Check sheet for the modelled part. Datum: model origin and axes. Units: mm. A direction names the side the tool comes from. Round coordinates to 2 decimals unless told otherwise and drop trailing zeros. Order: outer loops, then holes, each group sorted by start corner. A loop starts at its lowest first (then second) coordinate and runs counter-clockwise, first axis right, second up.
Autodesk Inventor part; units mm, degrees
ref_plane "YZ Plane" through (0, 0, 0) normal (1, 0, 0) x (0, 1, 0)
ref_plane "XZ Plane" through (0, 0, 0) normal (0, 1, 0) x (-1, 0, 0)
ref_plane "XY Plane" through (0, 0, 0) normal (0, 0, 1) x (1, 0, 0)
sketch "Sketch1" plane through (0, 0, 0) normal (0, 0, 1) x (1, 0, 0)
  circle A0 centre (0, 0) radius 17
  circle A1 centre (0, 0) radius 17.25
  circle A2 centre (0, 0) radius 4
  circle A3 centre (0, 0) radius 9
  circle A4 centre (0, 0) radius 2.5
  circle A5 centre (0, 6) radius 1.25
  dimension "d0" = 34
  dimension "d1" = 34.5
  dimension "d2" = 8
  dimension "d3" = 18
  dimension "d4" = 5
  dimension "d5" = 2.5
  dimension "d6" = 6
extrude "Extrusion1" add sketch "Sketch1" along normal blind 1 contours A1
extrude "Extrusion2" add sketch "Sketch1" along normal blind 3 contours A0
extrude "Extrusion3" add sketch "Sketch1" along normal blind 6 contours A3
extrude "Extrusion4" add sketch "Sketch1" along normal blind 15 contours A2
chamfer "Chamfer1" distance 0.2 angle 45 2 edges at (-17.25, 0, 0) (-17, 0, 3)
chamfer "Chamfer2" distance 0.1 angle 45 1 edges at (-2.5, 0, 15)
properties part number "HeatExchangePistonExhaust"
Item 1: Sectioned sample at A-A (y = 0). Record the cut outline in (x, z), and give its area (3 significant figures).
Answer:
outline: (-17.25, 0.2) - (-17.05, 0) - (-2.5, 0) - (-2.5, 14.9) - (-2.6, 15) - (-4, 15) - (-4, 6) - (-9, 6) - (-9, 3) - (-16.8, 3) - (-17, 2.8) - (-17, 1) - (-17.25, 1) - close; (2.5, 0) - (17.05, 0) - (17.25, 0.2) - (17.25, 1) - (17, 1) - (17, 2.8) - (16.8, 3) - (9, 3) - (9, 6) - (4, 6) - (4, 15) - (2.6, 15) - (2.5, 14.9) - close
area: 153 mm2
Item 2: Sectioned sample at B-B (x = 0). State how many separate pieces and enclosed holes the cut face has, and give its area (3 significant figures).
Answer:
separate pieces: 3
enclosed holes: 0
area: 138 mm2
Item 3: Go/stop test with flat-tipped pins: P1, Ø3, axis at x = 0, y = 0, coming from the -Z side; P2, Ø9, axis at x = 1, y = 1, coming from the +Z side; P3, Ø1.5, axis at x = -1, z = 6, coming from the -Y side. Record where each tip stops, or that it passes through.
Answer:
P1: passes through
P2: stops at z = 15
P3: stops at y = -9
Item 4: Sectioned sample at D-D (z = 10.25). Record the cut outline in (x, y), and give its area (3 significant figures).
Answer:
outline: circle Ø8 at (0, 0); hole circle Ø5 at (0, 0)
area: 30.6 mm2
Item 5: Scan lines: line 1 along Y through (x, z) = (0, 3.95); line 2 along Y through (x, z) = (0, 2.3); line 3 along Z through (x, y) = (-6.5, -7). Record each from-to range of solid material in increasing order.
Answer:
line 1: y = -9 to -2.5, 2.5 to 4.75, 7.25 to 9
line 2: y = -17 to -2.5, 2.5 to 4.75, 7.25 to 17
line 3: z = 0 to 3
Item 6: Access from +Z, -Z, +X, -X, +Y, -Y to the whole of each face (thin tool, end or side, straight path). Record for faces 4 (the cylindrical face through (-1.172, -8.923, 4.479)), 5 (the cylindrical face through (-0.54, 2.44, 7.35)).
Answer:
face 4: +Z
face 5: +Z, -Z
Item 7: Sectioned sample at C-C (z = 3.75). Record the cut outline in (x, y), and give its area (3 significant figures).
Answer:
outline: circle Ø18 at (0, 0); hole circle Ø5 at (0, 0); hole circle Ø2.5 at (0, 6)
area: 230 mm2
Item 8: Release check for a two-part mould opening along Y. For faces 1 (the flat face through (4, 0, 0)), 2 (the cylindrical face through (-0.867, 3.905, 10.437)), 3 (the cylindrical face through (-0.27, 7.22, 2.96)) record: released by +Y, released by -Y, zero draft, split by the parting line, or undercut.
Answer:
face 1: zero draft
face 2: split by the parting line
face 3: undercut
